```python
from build123d import *

# Parameters (mm, degrees)
SKETCH1_R           = 1.75
SKETCH1_R_2         = 1.25
BOSS_EXTRUDE1_DEPTH = 2
FILLET1_R           = 2


with BuildPart() as part:
    # Sketch1 → Boss-Extrude1 (new body)
    with BuildSketch(Plane(origin=(0, 0, 0), x_dir=(1, 0, 0), z_dir=(0, 1, 0))):
        with BuildLine():
            Line((-10609.380855774, 26644.275372767), (-10602.594176906, 26667.581570052))
            Line((-10602.594176906, 26667.581570052), (-10592.660823342, 26671.213057009))
            ThreePointArc((-10592.660823342, 26671.213057009), (-10588.813133366, 26669.425521878), (-10590.600668497, 26665.577831901))
            Line((-10590.600668497, 26665.577831901), (-10597.682341811, 26662.988877013))
            Line((-10597.682341811, 26662.988877013), (-10603.62012799, 26642.597870039))
            ThreePointArc((-10603.62012799, 26642.597870039), (-10607.339243246, 26640.556257511), (-10609.380855774, 26644.275372767))
        make_face()
        with Locations((-10591.63074592, 26668.395444455)):
            Circle(SKETCH1_R, mode=Mode.SUBTRACT)
        with Locations((-10600.138259358, 26665.285223533)):
            Circle(SKETCH1_R, mode=Mode.SUBTRACT)
        with Locations((-10606.500491882, 26643.436621403)):
            Circle(SKETCH1_R_2, mode=Mode.SUBTRACT)
    extrude(amount=BOSS_EXTRUDE1_DEPTH)

    # Fillet1
    fillet1_edges = [part.edges().sort_by_distance(p)[0] for p in [
        (-10597.682341811, 1, -26662.988877013),
        (-10602.594176906, 1, -26667.581570052),
    ]]
    fillet(fillet1_edges, radius=FILLET1_R)


solid = part.part
```
For this review, take the finished solid that the model builds, in its own axes (mm). Round coordinates to 2 decimals unless told otherwise and drop trailing zeros. Loops run counter-clockwise (first coordinate to the right, second up) from the corner with the lowest first, then second, coordinate; pieces in that order, holes last.
(1) We need section A-A (z = -26664). Give the boundary of the cut face in (x, y).
Returned:
outline: (-10603.64, 0) - (-10601.33, 0) - (-10601.33, 2) - (-10603.64, 2) - close; (-10598.95, 0) - (-10594.92, 0) - (-10594.92, 2) - (-10598.95, 2) - close
(2) We need section B-B (x = -10600.5). Give the boundary of the cut face in (y, z).
Returned:
outline: (0, -26668.35) - (2, -26668.35) - (2, -26667) - (0, -26667) - close; (0, -26663.57) - (2, -26663.57) - (2, -26653.31) - (0, -26653.31) - close
(3) We need section C-C (y = 0.75). Give the boundary of the cut face in (x, z), plus the area to 3 significant figures.
Returned:
outline: (-10609.38, -26644.28) - (-10602.88, -26666.61) arc R2 ccw to (-10601.64, -26667.93) - (-10592.66, -26671.21) arc R3 ccw to (-10590.6, -26665.58) - (-10596.73, -26663.34) arc R2 cw to (-10597.97, -26662.02) - (-10603.62, -26642.6) arc R3 ccw to start; hole circle Ø2.5 at (-10606.5, -26643.44); hole circle Ø3.5 at (-10600.14, -26665.29); hole circle Ø3.5 at (-10591.63, -26668.4)
area: 195 mm2
(4) We need section D-D (x = -10604). Give the boundary of the cut face in (y, z).
Returned:
outline: (0, -26662.75) - (2, -26662.75) - (2, -26641.78) - (0, -26641.78) - close
(5) Clearance check with a flat-ended pin moving along its axis: P1, Ø6, axis at x = -10596.5, z = -26651, coming from the +Y side. State where the tip first meets the part, or that it passes through.
Returned:
P1: passes through
(6) Wall thickness on line 1 along Z through (x, y) = (-10592, 1.2); line 2 along Z through (x, y) = (-10591.5, 1.9); line 3 along Z through (x, y) = (-10597.75, 1.85): over which ranges is each line inside the solid? List them lowest first.
Returned:
line 1: z = -26671.37 to -26670.11, -26666.68 to -26665.07
line 2: z = -26671.39 to -26670.14, -26666.65 to -26665.25
line 3: z = -26669.35 to -26662.5
(7) Mouldability with a two-part tool opening along Z and no side actions: class faces 1 (the cylindrical face through (-10605.308, 0.986, -26643.812)), 2 (the flat face through (-10606.175, 0.986, -26655.286)), 3 (the cylindrical face through (-10597.515, 1.014, -26662.814)) as released by +Z, released by -Z, zero draft, split by the parting line, or undercut.
Returned:
face 1: undercut
face 2: released by -Z
face 3: released by +Z
